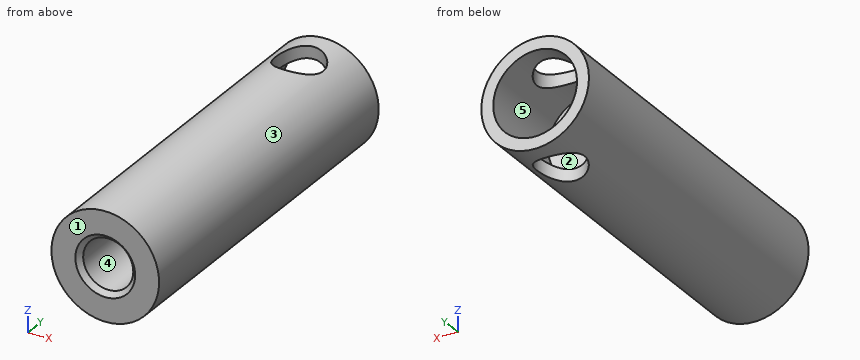
Autodesk Inventor part; units mm, degrees
ref_plane "YZ Plane" through (0, 0, 0) normal (1, 0, 0) x (0, 1, 0)
ref_plane "XZ Plane" through (0, 0, 0) normal (0, 1, 0) x (-1, 0, 0)
ref_plane "XY Plane" through (0, 0, 0) normal (0, 0, 1) x (1, 0, 0)
sketch "Sketch2" plane through (0, 0, 0) normal (0, 1, 0) x (-1, 0, 0)
  circle A0 centre (0, 0) radius 9
  dimension "d2" = 18
extrude "Extrusion2" add sketch "Sketch2" along normal blind 60
hole "Hole1" at (0, 0, 0) direction (0, 1, 0) diameter 8.376 depth 25 tip angle 118 countersink diameter 10 countersink angle 90
sketch "Sketch3" plane through (0, 60, 0) normal (0, 1, 0) x (1, 0, 0)
  point P0 (0, 0)
  point P1 (0, 0)
hole "Hole2" at (0, 60, 0) direction (0, -1, 0) diameter 14 depth 15 tip angle 118
sketch "Sketch4" plane through (0, 0, 0) normal (0, 0, 1) x (1, 0, 0)
  circle A0 centre (0, 53) radius 4
  line L0 (9, 60) -> (-9, 60)
  point P0 (0, 0)
  point P1 (0, 60)
  dimension "d20" = 8
  dimension "d21" = 7
extrude "Extrusion3" cut sketch "Sketch4" along normal through all both and the other way through all
sketch "Sketch5" plane through (0, 0, 0) normal (0, -1, 0) x (1, 0, 0)
  circle A0 centre (0, 0) radius 9
  line L0 (9, 0) -> (-9, 0)
  line L1 (-9, 0) -> (-9, -9)
  line L2 (-9, -9) -> (9, -9)
  line L3 (9, -9) -> (9, 0)
  dimension "d24" = 18
  dimension "d25" = 9
  dimension "d26" = 9
extrude "Extrusion4" [suppressed]
properties part number "RS-STT-103" material "11 110 (1.0721)"
The model under review builds one solid part; all positions refer to its coordinate system, in mm. Face numbers are marked on the shaded views. A direction names the side the tool comes from. Coordinates: 2 decimals unless noted, no trailing zeros. Loops run counter-clockwise (first coordinate to the right, second up) from the corner with the lowest first, then second, coordinate; pieces in that order, holes last.
(1) Consider section B-B, the plane y = 9. Give the boundary of the cut face in (x, z), plus the area to 3 significant figures.
Determined:
outline: circle Ø18 at (0, 0); hole circle Ø8.38 at (0, 0)
area: 199 mm2
(2) Consider section C-C, the plane x = 2.25. Give the number of separate pieces and of enclosed holes in the cut face, plus the area to 3 significant figures.
Determined:
separate pieces: 3
enclosed holes: 0
area: 614 mm2
(3) Insertion check: P1, Ø5, axis at y = 28.5, z = 6, coming from the +X side; P2, Ø2, axis at x = 3, y = 30.5, coming from the -Z side; P3, Ø9.5, axis at x = 0, z = 0, coming from the -Y side. Each pin has a flat end and moves straight along its axis. Give the tip position at first contact, or say it passes through.
Determined:
P1: stops at x = 8.29
P2: stops at z = -8.77
P3: stops at y = 0.25
(4) Consider section A-A, the plane y = 53. Give the boundary of the cut face in (x, z).
Determined:
outline: (-4, -8.06) - (-4, -5.74) arc R7 cw to (-4, 5.74) - (-4, 8.06) arc R9 ccw to start; (4, -8.06) arc R9 ccw to (4, 8.06) - (4, 5.74) arc R7 cw to (4, -5.74) - close
(5) Tool access review of the marked faces 4 and 5: name each direction out of +Z, -Z, +X, -X, +Y, -Y from which nothing blocks a thin tool from reaching the whole face with its end or side.
Determined:
face 4: -Y
face 5: +Y
(6) Draft analysis for pull direction X (two halves, no side actions). For the marked faces 1, 2 and 3, state which applies: +X half, -X half, draft (parallel to the pull), parting line (faces both ways), or undercut.
Determined:
face 1: draft
face 2: undercut
face 3: parting line
(7) Wall thickness on L1, parallel to Z at x = 0, y = 16.5; L2, parallel to Y at x = 0, z = 7.25; L3, parallel to Y at x = 2.5, z = 7: over which ranges is each line inside the solid? List them lowest first.
Determined:
L1: z = -9 to -4.19, 4.19 to 9
L2: y = 0 to 49, 57 to 60
L3: y = 0 to 49.88, 56.12 to 60
(8) Consider section D-D, the plane y = 38. Give the boundary of the cut face in (x, z), plus the area to 3 significant figures.
Determined:
outline: circle Ø18 at (0, 0)
area: 254 mm2
